Part model, mm, in its own coordinate system. Round coordinates to 2 decimals unless told otherwise and drop trailing zeros. Loops run counter-clockwise (first coordinate to the right, second up) from the corner with the lowest first, then second, coordinate; pieces in that order, holes last. Notation, with made-up numbers: M -31.5,-14.75 L 4.5,-14.75 A30 cw 4.5,15.25 Z; hole C 53,81 d9. An arc over 180 degrees is marked long. Put each result on its own line as item: value. Start each with the question number.
1) Probe line 1 along X through (y, z) = (2.05, -103.3) (3 decimals); line 2 along Z through (x, y) = (-59.5, 0.75); line 3 along X through (y, z) = (2.2, -55). List the from-to ranges inside material, lowest first.
2) Slice it at D-D on z = -93.6. Give the cut face in (x, y).
3) Slice it at A-A on x = -59.5. Give the cut face in (y, z), then the cut area to 4 significant figures.
4) Drop a flat-ended pin along its axis: pin 1 Ø3.5 at (x, z) = (-4.125, -103.3) entering from -Y. Give the stop position or say it passes through.
5) Pull direction Z, two halves, no side cores. Call faces 1 (the flat face through (-59, 1, 0)), 2 (the cylindrical face through (-2.98, 1.27, -3.33)), 3 (the flat face through (-19, 2.5, -54)): +Z half, -Z half, draft (parallel to the pull), parting line (faces both ways), or undercut.
6) Slice it at C-C on y = 1.35. State how many separate pieces and enclosed holes the cut face has, then the cut area to 3 significant figures.
7) Slice it at B-B on z = -55.15. Give the cut face in (x, y), then the cut area to 3 significant figures.
Autodesk Inventor part; units mm, degrees
ref_plane "Work Plane1" through (-59.5, 0, 0) normal (1, 0, 0) x (0, 0, -1)
ref_plane "YZ Plane" through (0, 0, 0) normal (1, 0, 0) x (0, 1, 0)
ref_plane "XZ Plane" through (0, 0, 0) normal (0, 1, 0) x (-1, 0, 0)
sketch "Sketch1" plane through (0, 0, 0) normal (0, 1, 0) x (-1, 0, 0)
  line L0 (0, 0) -> (119, 0)
  line L1 (119, 0) -> (119, -110.3)
  line L2 (119, -110.3) -> (0, -110.3)
  line L3 (0, -110.3) -> (0, 0)
  dimension "d0" = 119
  dimension "d1" = 110.3
extrude "Extrusion1" add sketch "Sketch1" along normal blind 2.5
sketch "Sketch2" plane through (0, 2.5, 0) normal (0, 1, 0) x (1, 0, 0)
  line L0 (-119, 0) -> (0, 0)
  line L1 (0, 0) -> (0, 110.3)
  line L2 (0, 110.3) -> (-119, 110.3)
  line L3 (-119, 110.3) -> (-119, 0)
  circle A0 centre (-114.875, 4.375) radius 1.55
  circle A1 centre (-114.875, 103.3) radius 1.55
  dimension "d4" = 3.1
  dimension "d5" = 4.125
  dimension "d6" = 4.375
  dimension "d7" = 3.1
  dimension "d8" = 7
extrude "Extrusion2" cut sketch "Sketch2" against normal blind 2.5 contours A0 | A1
ref_plane "Work Plane1" through (-59.5, 0, 0) normal (1, 0, 0) x (0, 0, -1)
mirror "Mirror1" about plane through (-59.5, 0, 0) normal (1, 0, 0) of "Extrusion2"
sketch "Sketch3" plane through (0, 2.5, 0) normal (0, 1, 0) x (1, 0, 0)
  circle A0 centre (-4.125, 4.375) radius 1.55
  circle A1 centre (-4.125, 103.3) radius 1.55
  circle A2 centre (-114.875, 4.375) radius 1.55
  circle A3 centre (-114.875, 103.3) radius 1.55
  line L0 (-119, 0) -> (0, 0)
  line L1 (0, 0) -> (0, 110.3)
  line L2 (0, 110.3) -> (-119, 110.3)
  line L3 (-119, 110.3) -> (-119, 0)
  circle A4 centre (-59.5, 55.15) radius 40
  circle A5 centre (-23.75, 19.4) radius 1.35
  circle A6 centre (-95.25, 19.4) radius 1.35
  circle A7 centre (-95.25, 93.6) radius 1.35
  circle A8 centre (-23.75, 93.6) radius 1.35
  dimension "d16" = 2.7
  dimension "d17" = 2.7
  dimension "d18" = 2.7
  dimension "d19" = 2.7
  dimension "d30" = 71.5
  dimension "d31" = 71.5
  dimension "d32" = 71.5
  dimension "d34" = 35.75
  dimension "d35" = 35.75
  dimension "d36" = 35.75
extrude "Extrusion3" cut sketch "Sketch3" against normal blind 2.5 contours A4 | A5 | A6 | A7 | A8
properties part number "Base Cover Right 6010 Fan"
Recorded:
1. line 1: x = -119 to -116.425, -113.325 to -5.675, -2.575 to 0
1. line 2: z = -110.3 to -95.15, -15.15 to 0
1. line 3: x = -119 to -99.5, -19.5 to 0
2. outline: M -119,0 L -96.6,0 L -96.6,2.5 L -119,2.5 Z; M -93.9,0 L -70.53,0 L -70.53,2.5 L -93.9,2.5 Z; M -48.47,0 L -25.1,0 L -25.1,2.5 L -48.47,2.5 Z; M -22.4,0 L 0,0 L 0,2.5 L -22.4,2.5 Z
3. outline: M 0,-110.3 L 2.5,-110.3 L 2.5,-95.15 L 0,-95.15 Z; M 0,-15.15 L 2.5,-15.15 L 2.5,0 L 0,0 Z
3. area: 75.75 mm2
4. pin 1: stops at y = 0
5. face 1: +Z half
5. face 2: undercut
5. face 3: draft
6. separate pieces: 1
6. enclosed holes: 9
6. area: 8,050 mm2
7. outline: M -119,0 L -99.5,0 L -99.5,2.5 L -119,2.5 Z; M -19.5,0 L 0,0 L 0,2.5 L -19.5,2.5 Z
7. area: 97.5 mm2
